```python
from build123d import *

# Parameters (mm, degrees)
SKETCH1_W            = 2.54
SKETCH1_H            = 2.54
BOSS_EXTRUDE3_DEPTH  = 5.588
BOSS_EXTRUDE4_START  = 5.588
BOSS_EXTRUDE4_DEPTH  = 73.66
BOSS_EXTRUDE6_START  = 79.248
SKETCH1_8_W          = 2.54
SKETCH1_8_H          = 2.54
SKETCH1_8_W_2        = 13.843
BOSS_EXTRUDE6_DEPTH  = 30.48
BOSS_EXTRUDE7_START  = 109.728
SKETCH1_9_W          = 12.7
SKETCH1_9_H          = 2.54
SKETCH1_9_W_2        = 2.54
SKETCH1_9_W_3        = 13.843
BOSS_EXTRUDE7_DEPTH  = 2.54
SKETCH4_W            = 50.546
SKETCH4_H            = 25.4
BOSS_EXTRUDE10_DEPTH = 2.54
FILLET1_R            = 1.905
SKETCH3_W            = 20.193
SKETCH3_H            = 5.08
CUT_EXTRUDE3_DEPTH   = 17.78


with BuildPart() as part:
    # Sketch1 → Boss-Extrude3 (new body)
    with BuildSketch(Plane(origin=(0, 0, 0), x_dir=(1, 0, 0), z_dir=(0, 1, 0))):
        with BuildLine():
            Line((-22.733, -10.16), (-22.733, -7.62))
            Line((-22.733, -7.62), (-22.733, 7.62))
            Line((-22.733, 7.62), (-5.08, 7.62))
            ThreePointArc((-5.08, 7.62), (-2.839806331, 9.489612663), (0, 10.16))
            Line((0, 10.16), (-25.273, 10.16))
            Line((-25.273, 10.16), (-25.273, -10.16))
            Line((-25.273, -10.16), (-22.733, -10.16))
        make_face()
        with BuildLine():
            ThreePointArc((0, 10.16), (2.839806331, 9.489612663), (5.08, 7.62))
            Line((5.08, 7.62), (22.733, 7.62))
            Line((22.733, 7.62), (22.733, -7.62))
            Line((22.733, -7.62), (22.733, -10.16))
            Line((22.733, -10.16), (25.273, -10.16))
            Line((25.273, -10.16), (25.273, 10.16))
            Line((25.273, 10.16), (0, 10.16))
        make_face()
        with BuildLine():
            ThreePointArc((0, 10.16), (-2.839806331, 9.489612663), (-5.08, 7.62))
            Line((-5.08, 7.62), (5.08, 7.62))
            ThreePointArc((5.08, 7.62), (2.839806331, 9.489612663), (0, 10.16))
        make_face()
        with BuildLine():
            Line((-22.733, 7.62), (-22.733, -7.62))
            Line((-22.733, -7.62), (-20.193, -7.62))
            Line((-20.193, -7.62), (-20.193, -5.08))
            Line((-20.193, -5.08), (-20.193, 5.08))
            Line((-20.193, 5.08), (-6.221703947, 5.08))
            ThreePointArc((-6.221703947, 5.08), (-5.791806974, 6.413357827), (-5.08, 7.62))
            Line((-5.08, 7.62), (-22.733, 7.62))
        make_face()
        with Locations((-21.463, -8.89)):
            Rectangle(SKETCH1_W, SKETCH1_H)
        with BuildLine():
            Line((5.08, 7.62), (-5.08, 7.62))
            ThreePointArc((-5.08, 7.62), (-5.791806974, 6.413357827), (-6.221703947, 5.08))
            Line((-6.221703947, 5.08), (6.221703947, 5.08))
            ThreePointArc((6.221703947, 5.08), (5.791806974, 6.413357827), (5.08, 7.62))
        make_face()
        with BuildLine():
            Line((22.733, 7.62), (5.08, 7.62))
            ThreePointArc((5.08, 7.62), (5.791806974, 6.413357827), (6.221703947, 5.08))
            Line((6.221703947, 5.08), (20.193, 5.08))
            Line((20.193, 5.08), (20.193, -5.08))
            Line((20.193, -5.08), (20.193, -7.62))
            Line((20.193, -7.62), (22.733, -7.62))
            Line((22.733, -7.62), (22.733, 7.62))
        make_face()
        with Locations((21.463, -8.89)):
            Rectangle(SKETCH1_W, SKETCH1_H)
    extrude(amount=BOSS_EXTRUDE3_DEPTH)

    # Sketch1<7> → Boss-Extrude4 (add)
    with BuildSketch(Plane(origin=(0, 0, 0), x_dir=(1, 0, 0), z_dir=(0, 1, 0)).offset(BOSS_EXTRUDE4_START)):
        with BuildLine():
            Line((-22.733, -10.16), (-22.733, -7.62))
            Line((-22.733, -7.62), (-22.733, 7.62))
            Line((-22.733, 7.62), (-5.08, 7.62))
            ThreePointArc((-5.08, 7.62), (-2.839806331, 9.489612663), (0, 10.16))
            Line((0, 10.16), (-25.273, 10.16))
            Line((-25.273, 10.16), (-25.273, -10.16))
            Line((-25.273, -10.16), (-22.733, -10.16))
        make_face()
        with BuildLine():
            ThreePointArc((0, 10.16), (2.839806331, 9.489612663), (5.08, 7.62))
            Line((5.08, 7.62), (22.733, 7.62))
            Line((22.733, 7.62), (22.733, -7.62))
            Line((22.733, -7.62), (22.733, -10.16))
            Line((22.733, -10.16), (25.273, -10.16))
            Line((25.273, -10.16), (25.273, 10.16))
            Line((25.273, 10.16), (0, 10.16))
        make_face()
        with BuildLine():
            ThreePointArc((0, 10.16), (-2.839806331, 9.489612663), (-5.08, 7.62))
            Line((-5.08, 7.62), (5.08, 7.62))
            ThreePointArc((5.08, 7.62), (2.839806331, 9.489612663), (0, 10.16))
        make_face()
    extrude(amount=BOSS_EXTRUDE4_DEPTH)

    # Sketch1<8> → Boss-Extrude6 (add)
    with BuildSketch(Plane(origin=(0, 0, 0), x_dir=(1, 0, 0), z_dir=(0, 1, 0)).offset(BOSS_EXTRUDE6_START)):
        with BuildLine():
            Line((-22.733, -10.16), (-22.733, -7.62))
            Line((-22.733, -7.62), (-22.733, 7.62))
            Line((-22.733, 7.62), (-5.08, 7.62))
            ThreePointArc((-5.08, 7.62), (-2.839806331, 9.489612663), (0, 10.16))
            Line((0, 10.16), (-25.273, 10.16))
            Line((-25.273, 10.16), (-25.273, -10.16))
            Line((-25.273, -10.16), (-22.733, -10.16))
        make_face()
        with BuildLine():
            Line((-22.733, 7.62), (-22.733, -7.62))
            Line((-22.733, -7.62), (-20.193, -7.62))
            Line((-20.193, -7.62), (-20.193, -5.08))
            Line((-20.193, -5.08), (-20.193, 5.08))
            Line((-20.193, 5.08), (-6.221703947, 5.08))
            ThreePointArc((-6.221703947, 5.08), (-5.791806974, 6.413357827), (-5.08, 7.62))
            Line((-5.08, 7.62), (-22.733, 7.62))
        make_face()
        with BuildLine():
            Line((-20.193, -5.08), (-20.193, -7.62))
            Line((-20.193, -7.62), (-6.35, -7.62))
            Line((-6.35, -7.62), (-6.35, -3.175))
            Line((-6.35, -3.175), (-6.35, 3.81))
            ThreePointArc((-6.35, 3.81), (-6.317844572, 4.448231909), (-6.221703947, 5.08))
            Line((-6.221703947, 5.08), (-20.193, 5.08))
            Line((-20.193, 5.08), (-20.193, -5.08))
        make_face()
        with Locations((-21.463, -8.89)):
            Rectangle(SKETCH1_8_W, SKETCH1_8_H)
        with Locations((-13.2715, -8.89)):
            Rectangle(SKETCH1_8_W_2, SKETCH1_8_H)
        with BuildLine():
            ThreePointArc((0, 10.16), (2.839806331, 9.489612663), (5.08, 7.62))
            Line((5.08, 7.62), (22.733, 7.62))
            Line((22.733, 7.62), (22.733, -7.62))
            Line((22.733, -7.62), (22.733, -10.16))
            Line((22.733, -10.16), (25.273, -10.16))
            Line((25.273, -10.16), (25.273, 10.16))
            Line((25.273, 10.16), (0, 10.16))
        make_face()
        with BuildLine():
            Line((22.733, 7.62), (5.08, 7.62))
            ThreePointArc((5.08, 7.62), (5.791806974, 6.413357827), (6.221703947, 5.08))
            Line((6.221703947, 5.08), (20.193, 5.08))
            Line((20.193, 5.08), (20.193, -5.08))
            Line((20.193, -5.08), (20.193, -7.62))
            Line((20.193, -7.62), (22.733, -7.62))
            Line((22.733, -7.62), (22.733, 7.62))
        make_face()
        with BuildLine():
            Line((6.35, -3.175), (6.35, -7.62))
            Line((6.35, -7.62), (20.193, -7.62))
            Line((20.193, -7.62), (20.193, -5.08))
            Line((20.193, -5.08), (20.193, 5.08))
            Line((20.193, 5.08), (6.221703947, 5.08))
            ThreePointArc((6.221703947, 5.08), (6.317844572, 4.448231909), (6.35, 3.81))
            Line((6.35, 3.81), (6.35, -3.175))
        make_face()
        with Locations((13.2715, -8.89)):
            Rectangle(SKETCH1_8_W_2, SKETCH1_8_H)
        with Locations((21.463, -8.89)):
            Rectangle(SKETCH1_8_W, SKETCH1_8_H)
        with BuildLine():
            ThreePointArc((0, 10.16), (-2.839806331, 9.489612663), (-5.08, 7.62))
            Line((-5.08, 7.62), (5.08, 7.62))
            ThreePointArc((5.08, 7.62), (2.839806331, 9.489612663), (0, 10.16))
        make_face()
    extrude(amount=BOSS_EXTRUDE6_DEPTH)

    # Sketch1<9> → Boss-Extrude7 (add)
    with BuildSketch(Plane(origin=(0, 0, 0), x_dir=(1, 0, 0), z_dir=(0, 1, 0)).offset(BOSS_EXTRUDE7_START)):
        with BuildLine():
            Line((-6.35, -3.175), (-6.35, -7.62))
            Line((-6.35, -7.62), (6.35, -7.62))
            Line((6.35, -7.62), (6.35, -3.175))
            Line((6.35, -3.175), (6.35, 3.81))
            ThreePointArc((6.35, 3.81), (6.317844572, 4.448231909), (6.221703947, 5.08))
            Line((6.221703947, 5.08), (-6.221703947, 5.08))
            ThreePointArc((-6.221703947, 5.08), (-6.317844572, 4.448231909), (-6.35, 3.81))
            Line((-6.35, 3.81), (-6.35, -3.175))
        make_face()
        with Locations((0, -8.89)):
            Rectangle(SKETCH1_9_W, SKETCH1_9_H)
        with BuildLine():
            Line((5.08, 7.62), (-5.08, 7.62))
            ThreePointArc((-5.08, 7.62), (-5.791806974, 6.413357827), (-6.221703947, 5.08))
            Line((-6.221703947, 5.08), (6.221703947, 5.08))
            ThreePointArc((6.221703947, 5.08), (5.791806974, 6.413357827), (5.08, 7.62))
        make_face()
        with BuildLine():
            Line((-22.733, -10.16), (-22.733, -7.62))
            Line((-22.733, -7.62), (-22.733, 7.62))
            Line((-22.733, 7.62), (-5.08, 7.62))
            ThreePointArc((-5.08, 7.62), (-2.839806331, 9.489612663), (0, 10.16))
            Line((0, 10.16), (-25.273, 10.16))
            Line((-25.273, 10.16), (-25.273, -10.16))
            Line((-25.273, -10.16), (-22.733, -10.16))
        make_face()
        with Locations((-21.463, -8.89)):
            Rectangle(SKETCH1_9_W_2, SKETCH1_9_H)
        with BuildLine():
            Line((-22.733, 7.62), (-22.733, -7.62))
            Line((-22.733, -7.62), (-20.193, -7.62))
            Line((-20.193, -7.62), (-20.193, -5.08))
            Line((-20.193, -5.08), (-20.193, 5.08))
            Line((-20.193, 5.08), (-6.221703947, 5.08))
            ThreePointArc((-6.221703947, 5.08), (-5.791806974, 6.413357827), (-5.08, 7.62))
            Line((-5.08, 7.62), (-22.733, 7.62))
        make_face()
        with Locations((-13.2715, -8.89)):
            Rectangle(SKETCH1_9_W_3, SKETCH1_9_H)
        with BuildLine():
            Line((-20.193, -5.08), (-20.193, -7.62))
            Line((-20.193, -7.62), (-6.35, -7.62))
            Line((-6.35, -7.62), (-6.35, -3.175))
            Line((-6.35, -3.175), (-6.35, 3.81))
            ThreePointArc((-6.35, 3.81), (-6.317844572, 4.448231909), (-6.221703947, 5.08))
            Line((-6.221703947, 5.08), (-20.193, 5.08))
            Line((-20.193, 5.08), (-20.193, -5.08))
        make_face()
        with BuildLine():
            ThreePointArc((0, 10.16), (-2.839806331, 9.489612663), (-5.08, 7.62))
            Line((-5.08, 7.62), (5.08, 7.62))
            ThreePointArc((5.08, 7.62), (2.839806331, 9.489612663), (0, 10.16))
        make_face()
        with BuildLine():
            Line((22.733, 7.62), (5.08, 7.62))
            ThreePointArc((5.08, 7.62), (5.791806974, 6.413357827), (6.221703947, 5.08))
            Line((6.221703947, 5.08), (20.193, 5.08))
            Line((20.193, 5.08), (20.193, -5.08))
            Line((20.193, -5.08), (20.193, -7.62))
            Line((20.193, -7.62), (22.733, -7.62))
            Line((22.733, -7.62), (22.733, 7.62))
        make_face()
        with BuildLine():
            ThreePointArc((0, 10.16), (2.839806331, 9.489612663), (5.08, 7.62))
            Line((5.08, 7.62), (22.733, 7.62))
            Line((22.733, 7.62), (22.733, -7.62))
            Line((22.733, -7.62), (22.733, -10.16))
            Line((22.733, -10.16), (25.273, -10.16))
            Line((25.273, -10.16), (25.273, 10.16))
            Line((25.273, 10.16), (0, 10.16))
        make_face()
        with BuildLine():
            Line((6.35, -3.175), (6.35, -7.62))
            Line((6.35, -7.62), (20.193, -7.62))
            Line((20.193, -7.62), (20.193, -5.08))
            Line((20.193, -5.08), (20.193, 5.08))
            Line((20.193, 5.08), (6.221703947, 5.08))
            ThreePointArc((6.221703947, 5.08), (6.317844572, 4.448231909), (6.35, 3.81))
            Line((6.35, 3.81), (6.35, -3.175))
        make_face()
        with Locations((13.2715, -8.89)):
            Rectangle(SKETCH1_9_W_3, SKETCH1_9_H)
        with Locations((21.463, -8.89)):
            Rectangle(SKETCH1_9_W_2, SKETCH1_9_H)
    extrude(amount=BOSS_EXTRUDE7_DEPTH)

    # Sketch4 → Boss-Extrude10 (add)
    with BuildSketch(Plane.XY.offset(10.16)):
        with Locations((0, 12.7)):
            Rectangle(SKETCH4_W, SKETCH4_H)
    extrude(amount=BOSS_EXTRUDE10_DEPTH)

    # Fillet1
    fillet1_edges = [part.edges().sort_by_distance(p)[0] for p in [
        (-25.273, 25.4, 11.43),
        (25.273, 25.4, 11.43),
        (-25.273, 12.7, 12.7),
        (25.273, 12.7, 12.7),
        (-25.273, 0, 1.27),
        (0, 0, -10.16),
        (25.273, 0, 1.27),
        (-25.273, 68.834, 10.16),
        (-25.273, 56.134, -10.16),
        (25.273, 56.134, -10.16),
        (25.273, 68.834, 10.16),
        (0, 112.268, 10.16),
        (25.273, 112.268, 0),
        (-25.273, 112.268, 0),
        (0, 112.268, -10.16),
    ]]
    fillet(fillet1_edges, radius=FILLET1_R)

    # Sketch3 → Cut-Extrude3 (cut)
    with BuildSketch(Plane.XY.offset(10.16)):
        with Locations((-15.1765, 107.188)):
            Rectangle(SKETCH3_W, SKETCH3_H)
    extrude(amount=-CUT_EXTRUDE3_DEPTH, mode=Mode.SUBTRACT)


solid = part.part
```
Work out the finished part from the listing and answer in its coordinate system (mm). A direction names the side the tool comes from. Give positions to 0.01 mm unless a question says otherwise; leave off trailing zeros. Write each loop counter-clockwise with the first axis right and the second up, starting at its lowest first coordinate (ties: lowest second). Pieces come first, ordered by that corner, then holes. Notation, with made-up numbers: (-20.75, 37) -> (35.25, 37) arc R34 cw to (35.25, 67) -> close; hole circle Ø3 at (21, 57.5). An arc over 180 degrees is marked (long way). Write each question's results on one line, items separated by ' | '.
1. Straight lines are drawn through the part: L1, parallel to Y at x = -12.5, z = -5.5; L2, parallel to X at y = 40, z = -3.5; L3, parallel to Z at x = -3.5, y = 8. For each, find the intervals that lie inside material, in ascending order.
Data:
L1: 0 to 5.59, 79.25 to 104.65, 109.73 to 112.27 | L2: -25.27 to -22.73, 22.73 to 25.27 | L3: -10.16 to -7.62, 10.16 to 12.7
2. Find section B-B on x = -14.5. Determine the outline of the cut face in (y, z) (3 decimals).
Data:
outline: (0, -8.255) arc R1.905 ccw to (1.905, -10.16) -> (110.363, -10.16) arc R1.905 ccw to (112.268, -8.255) -> (112.268, 8.255) arc R1.905 ccw to (110.363, 10.16) -> (109.728, 10.16) -> (109.728, -7.62) -> (104.648, -7.62) -> (104.648, 10.16) -> (79.248, 10.16) -> (79.248, -7.62) -> (5.588, -7.62) -> (5.588, -5.08) -> (0, -5.08) -> close; (0, 10.16) -> (25.4, 10.16) -> (25.4, 12.7) -> (0, 12.7) -> close
3. Each of these flat-tipped pins is pushed along its axis until it touches: pin 1 Ø4 at (x, y) = (16.5, 75.5) entering from +Z; pin 2 Ø1.5 at (x, z) = (1.5, 0.5) entering from -Y; pin 3 Ø1 at (x, z) = (17.5, 8) entering from -Y. Where does it stop, or does it pass through?
Data:
pin 1: z = -7.62 | pin 2: y = 109.73 | pin 3: y = 79.25
4. Find section C-C on y = 98. Determine the outline of the cut face in (x, z) (3 decimals).
Data:
outline: (-25.273, -8.255) arc R1.905 ccw to (-23.368, -10.16) -> (23.368, -10.16) arc R1.905 ccw to (25.273, -8.255) -> (25.273, 8.255) arc R1.905 ccw to (23.368, 10.16) -> (6.35, 10.16) -> (6.35, -3.81) arc R6.35 cw to (5.08, -7.62) -> (-5.08, -7.62) arc R6.35 cw to (-6.35, -3.81) -> (-6.35, 10.16) -> (-23.368, 10.16) arc R1.905 ccw to (-25.273, 8.255) -> close
5. Determine the mould class of faces 1 (the flat face through (-2, 47, -7.62)), 2 (the cylindrical face through (-24.73, 63.503, 9.587)), 3 (the cylindrical face through (24.73, 24.827, 11.003)) for opening direction Z: +Z half, -Z half, draft (parallel to the pull), parting line (faces both ways), or undercut.
Data:
face 1: undercut | face 2: +Z half | face 3: draft
6. Find section A-A on z = -0.25. Determine the outline of the cut face in (x, y) (3 decimals).
Data:
outline: (-25.273, 1.905) arc R1.905 ccw to (-23.368, 0) -> (-20.193, 0) -> (-20.193, 5.588) -> (-22.733, 5.588) -> (-22.733, 79.248) -> (-6.35, 79.248) -> (-6.35, 104.648) -> (-25.273, 104.648) -> close; (-25.273, 109.728) -> (6.35, 109.728) -> (6.35, 79.248) -> (22.733, 79.248) -> (22.733, 5.588) -> (20.193, 5.588) -> (20.193, 0) -> (23.368, 0) arc R1.905 ccw to (25.273, 1.905) -> (25.273, 110.363) arc R1.905 ccw to (23.368, 112.268) -> (-23.368, 112.268) arc R1.905 ccw to (-25.273, 110.363) -> close
7. Find section D-D on x = 9. Determine the outline of the cut face in (y, z) (3 decimals).
Data:
outline: (0, -8.255) arc R1.905 ccw to (1.905, -10.16) -> (110.363, -10.16) arc R1.905 ccw to (112.268, -8.255) -> (112.268, 8.255) arc R1.905 ccw to (110.363, 10.16) -> (79.248, 10.16) -> (79.248, -7.62) -> (5.588, -7.62) -> (5.588, -5.08) -> (0, -5.08) -> close; (0, 10.16) -> (25.4, 10.16) -> (25.4, 12.7) -> (0, 12.7) -> close
8. A tool of negligible diameter and unlimited length cuts with its end or side. For faces 4 (the flat face through (-15, 104.648, 1)), 5 (the flat face through (-16, 88, 10.16)), 6 (the cylindrical face through (24.73, 66.321, 9.587)), from which of +Z, -Z, +X, -X, +Y, -Y can it reach the whole face along a straight path? Write none if from no direction.
Data:
face 4: +Z, -X | face 5: +Z, +X, -X, +Y | face 6: +Z, +X, +Y
